Could you check a few things on this model? Use its own coordinates, in mm. Face numbers are marked on the shaded views. A direction names the side the tool comes from. Coordinates: 2 decimals unless noted, no trailing zeros. Order: outer loops, then holes, each group sorted by start corner. A loop starts at its lowest first (then second) coordinate and runs counter-clockwise, first axis right, second up. Notation, with made-up numbers: (56.5, 48.25) -> (77.5, 48.25) arc R12 cw to (77.5, 62.25) -> close; hole circle Ø8 at (41, 86). An arc over 180 degrees is marked (long way). Return JSON: item names as keys, results as strings. Group by question number.
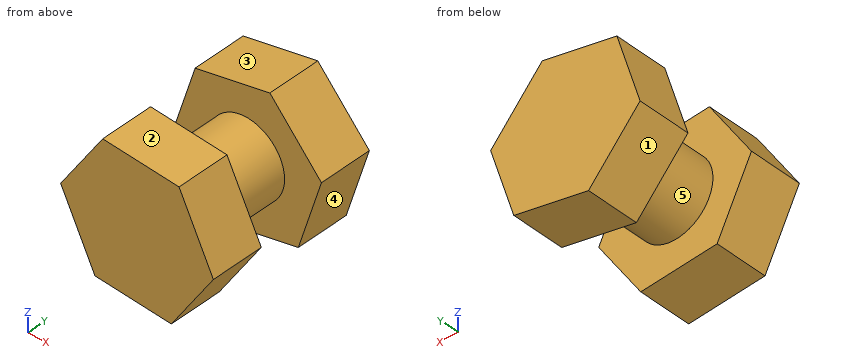
from build123d import *

# Parameters (mm, degrees)
SKETCH1_R           = 3.175
BOSS_EXTRUDE1_DEPTH = 10
BOSS_EXTRUDE2_DEPTH = 4.365625
BOSS_EXTRUDE3_DEPTH = 4.365625


with BuildPart() as part:
    # Sketch1 → Boss-Extrude1 (new body)
    with BuildSketch(Plane(origin=(0, 0, 0), x_dir=(1, 0, 0), z_dir=(0, 1, 0))):
        Circle(SKETCH1_R)
    extrude(amount=BOSS_EXTRUDE1_DEPTH)

    # Sketch2 → Boss-Extrude2 (add)
    with BuildSketch(Plane.XZ):
        Polygon((6.404947556, -0.373093671), (3.525582375, 5.360300458), (-2.879365181, 5.733394129), (-6.404947556, 0.373093671), (-3.525582375, -5.360300458), (2.879365181, -5.733394129), align=None)
    extrude(amount=BOSS_EXTRUDE2_DEPTH)

    # Sketch3 → Boss-Extrude3 (add)
    with BuildSketch(Plane(origin=(0, 10, 0), x_dir=(1, 0, 0), z_dir=(0, 1, 0))):
        Polygon((-6.266509765, 1.376011426), (-4.324915734, -4.738950937), (1.941594032, -6.114962363), (6.266509765, -1.376011426), (4.324915734, 4.738950937), (-1.941594032, 6.114962363), align=None)
    extrude(amount=-BOSS_EXTRUDE3_DEPTH)


solid = part.part
Q1. I want a section at A-A on z = 4.5. Please give me the cut outline in (x, y).
Q2. On a 3-axis mill with a long thin cutter (end or side, diameter ignored), from which of +Z, -Z, +X, -X, +Y, -Y can I reach the whole of each face in a straight line? I mean the marked faces 1, 2, 3, 4 and 5. Say none if no direction works.
Q3. I want a section at C-C on z = 1.75. Please give me the cut outline in (x, y), and give its area (3 significant figures).
Q4. I need wall thicknesses on line 1 along Y through (x, z) = (-0.75, -3.25); line 2 along Y through (x, z) = (5.75, 1.25); line 3 along X through (y, z) = (-1.5, -3.75). Which ranges of each line are inside material? Lowest first, please. Write a range as from..to.
Q5. I want a section at D-D on x = 0. Please give me the cut outline in (y, z) (3 decimals), and give its area (3 significant figures).
Q6. I want a section at B-B on y = -2.75. Please give me the cut outline in (x, z), and give its area (3 significant figures).
Q7. I'm going to push flat-ended pins straight in: pin 1 Ø3 at (x, y) = (4, 0) entering from -Z; pin 2 Ø3 at (x, y) = (-0.5, 3) entering from +Z (3 decimals); pin 3 Ø3 at (x, y) = (2.5, 2) entering from -Z. Where does each tip first touch, or does it pass through?
Response values:
{
 "1": {"outline": "(-4.4, 5.63) -> (3.42, 5.63) -> (3.42, 10) -> (-4.4, 10) -> close; (-3.69, -4.37) -> (3.96, -4.37) -> (3.96, 0) -> (-3.69, 0) -> close"},
 "2": {"face 1": "-Z, -X, +Y", "face 2": "+Z, +X, -Y", "face 3": "+Z, -X, +Y", "face 4": "-Z, +X, +Y", "face 5": "none"},
 "3": {"outline": "(-5.5, -4.37) -> (5.34, -4.37) -> (5.34, 0) -> (2.65, 0) -> (2.65, 5.63) -> (5.93, 5.63) -> (5.93, 10) -> (-5.27, 10) -> (-5.27, 5.63) -> (-2.65, 5.63) -> (-2.65, 0) -> (-5.5, 0) -> close", "area": "126 mm²"},
 "4": {"line 1": "y = -4.37..0, 5.63..10", "line 2": "y = 5.63..10", "line 3": "x = -4.33..4.18"},
 "5": {"outline": "(-4.366, -5.566) -> (0, -5.566) -> (0, -3.175) -> (5.634, -3.175) -> (5.634, -5.689) -> (10, -5.689) -> (10, 5.689) -> (5.634, 5.689) -> (5.634, 3.175) -> (0, 3.175) -> (0, 5.566) -> (-4.366, 5.566) -> close", "area": "134 mm²"},
 "6": {"outline": "(-6.4, 0.37) -> (-3.53, -5.36) -> (2.88, -5.73) -> (6.4, -0.37) -> (3.53, 5.36) -> (-2.88, 5.73) -> close", "area": "107 mm²"},
 "7": {"pin 1": "stops at z = -5.73", "pin 2": "stops at z = 3.175", "pin 3": "stops at z = -3.01"}
}
